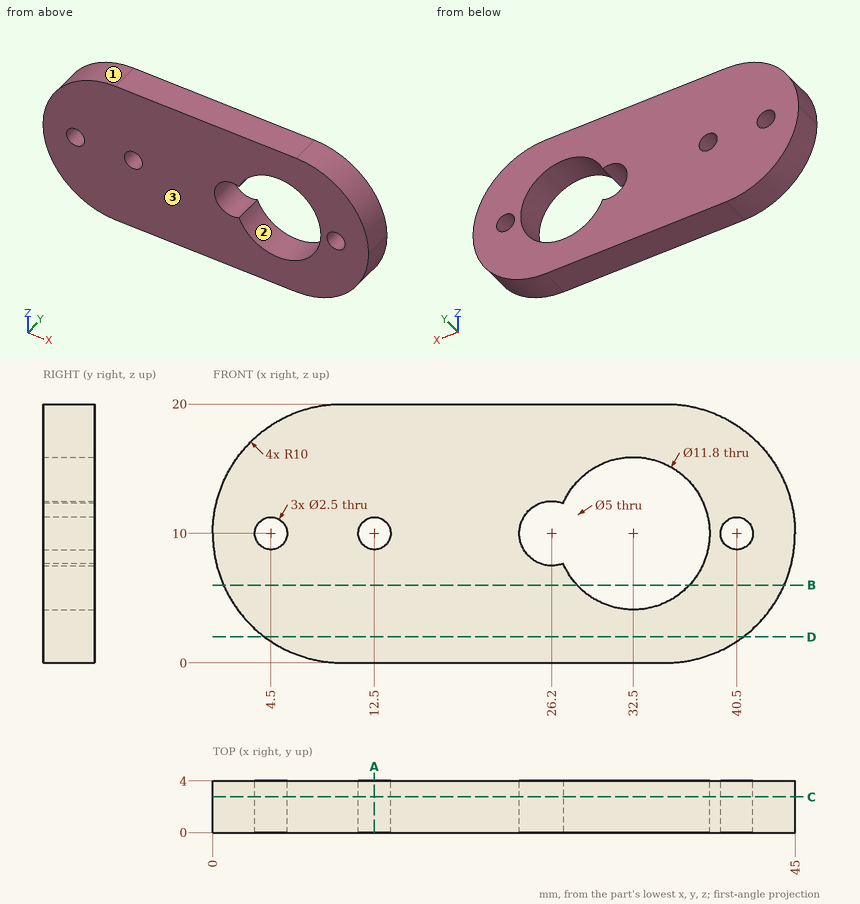
Drawing for the job (mm, zero at the part's lowest x, y, z). Round coordinates to 2 decimals unless told otherwise and drop trailing zeros. Write each loop counter-clockwise with the first axis right and the second up, starting at its lowest first coordinate (ties: lowest second). Pieces come first, ordered by that corner, then holes. Notation, with made-up numbers: M 10.25,-6 L 66.25,-6 A16 cw 66.25,22 Z; hole C 36.25,44.5 d3. An arc over 180 degrees is marked long. Put each result on its own line as item: value.
Item 1: Flat gauge pins, fed straight in: P1, Ø1, axis at y = 2.5, z = 7.5, coming from the -X side; P2, Ø1.5, axis at x = 4.5, z = 10, coming from the +Y side; P3, Ø1.5, axis at y = 3.5, z = 11.5, coming from the +X side; P4, Ø2, axis at x = 5.5, y = 0.5, coming from the +Z side. Where does each tip first touch, or does it go through?
Responses:
P1: x = 0.2
P2: through
P3: x = 44.97
P4: z = 19.37
Item 2: Cut at A-A (x = 12.5). List the corners of the cut face in (y, z).
Responses:
outline: M 0,0 L 4,0 L 4,8.75 L 0,8.75 Z; M 0,11.25 L 4,11.25 L 4,20 L 0,20 Z
Item 3: Mould opens along Z. For the marked faces 1, 2 and 3 say: +Z half, -Z half, draft (parallel to the pull), parting line (faces both ways), or undercut.
Responses:
face 1: +Z half
face 2: undercut
face 3: draft
Item 4: Cut at C-C (y = 2.75). State how many separate pieces and enclosed holes the cut face has, and give its area (3 significant figures).
Responses:
separate pieces: 1
enclosed holes: 4
area: 677 mm²
Item 5: Cut at D-D (z = 2). List the corners of the cut face in (x, y).
Responses:
outline: M 4,0 L 41,0 L 41,4 L 4,4 Z
Item 6: Probe L1, parallel to X at y = 2.7, z = 10; L2, parallel to Z at x = 32.5, y = 2.7; L3, parallel to Z at x = 26.2, y = 2.4. List the from-to ranges inside material, lowest first. Write a range as from..to.
Responses:
L1: 0..3.25, 5.75..11.25, 13.75..23.7, 38.4..39.25, 41.75..45
L2: 0..4.1, 15.9..20
L3: 0..7.5, 12.5..20
Item 7: Cut at B-B (z = 6). List the corners of the cut face in (x, y) (3 decimals), and give its area (3 significant figures).
Responses:
outline: M 0.835,0 L 28.163,0 L 28.163,4 L 0.835,4 Z; M 36.837,0 L 44.165,0 L 44.165,4 L 36.837,4 Z
area: 139 mm²
